Could you check a few things on this model? Use its own coordinates, in mm. A direction names the side the tool comes from. Give positions to 0.01 mm unless a question says otherwise; leave off trailing zeros. Order: outer loops, then holes, each group sorted by start corner. A loop starts at its lowest first (then second) coordinate and runs counter-clockwise, first axis right, second up. Notation, with made-up numbers: (-29, 57) -> (-20, 57) arc R17 cw to (-20, 81) -> close; hole circle Ø4 at (80.25, 41.5). An arc over 180 degrees is marked (long way). Use one line per item in the form item = value. Start each with the question number.
from build123d import *

# Parameters (mm, degrees)
SKETCH1_W           = 66
SKETCH1_H           = 33
SKETCH1_W_2         = 33
BOSS_EXTRUDE1_DEPTH = 100
SKETCH3_W           = 86
SKETCH3_H           = 86
CUT_EXTRUDE1_DEPTH  = 90
CUT_EXTRUDE2_DEPTH  = 2.5
CUT_EXTRUDE3_DEPTH  = 18.5
SKETCH6_W           = 120.471409441
SKETCH6_H           = 36
CUT_EXTRUDE4_DEPTH  = 5
CUT_EXTRUDE5_DEPTH  = 2.5
CUT_EXTRUDE6_DEPTH  = 10
SKETCH9_W           = 60
SKETCH9_H           = 10
CUT_EXTRUDE7_DEPTH  = 5
SKETCH10_W          = 40
SKETCH10_H          = 10
CUT_EXTRUDE8_DEPTH  = 5
SKETCH11_W          = 50
SKETCH11_H          = 50
CUT_EXTRUDE11_DEPTH = 3
CUT_EXTRUDE12_DEPTH = 10


with BuildPart() as part:
    # Sketch1 → Boss-Extrude1 (new body)
    with BuildSketch(Plane.XY):
        with BuildLine():
            Line((15, 0), (91, 0))
            ThreePointArc((91, 0), (101.606601718, 4.393398282), (106, 15))
            Line((106, 15), (106, 91))
            ThreePointArc((106, 91), (101.606601718, 101.606601718), (91, 106))
            Line((91, 106), (15, 106))
            ThreePointArc((15, 106), (4.393398282, 101.606601718), (0, 91))
            Line((0, 91), (0, 15))
            ThreePointArc((0, 15), (4.393398282, 4.393398282), (15, 0))
        make_face()
        with Locations((53, 31.5)):
            Rectangle(SKETCH1_W, SKETCH1_H, mode=Mode.SUBTRACT)
        with Locations((31.5, 69.5)):
            Rectangle(SKETCH1_W_2, SKETCH1_H, mode=Mode.SUBTRACT)
        with Locations((74.5, 69.5)):
            Rectangle(SKETCH1_W_2, SKETCH1_H, mode=Mode.SUBTRACT)
    extrude(amount=-BOSS_EXTRUDE1_DEPTH)

    # Sketch3 → Cut-Extrude1 (cut)
    with BuildSketch(Plane(origin=(0, 0, -100), x_dir=(-1, 0, 0), z_dir=(0, 0, -1))):
        with Locations((-53, 53)):
            Rectangle(SKETCH3_W, SKETCH3_H)
    extrude(amount=-CUT_EXTRUDE1_DEPTH, mode=Mode.SUBTRACT)

    # Sketch4 → Cut-Extrude2 (cut)
    with BuildSketch(Plane(origin=(0, 106, 0), x_dir=(1, 0, 0), z_dir=(0, 1, 0))):
        with BuildLine():
            Line((45, 43), (61, 43))
            ThreePointArc((61, 43), (62.414213562, 42.414213562), (63, 41))
            Line((63, 41), (63, 17))
            ThreePointArc((63, 17), (62.414213562, 15.585786438), (61, 15))
            Line((61, 15), (45, 15))
            ThreePointArc((45, 15), (43.585786438, 15.585786438), (43, 17))
            Line((43, 17), (43, 41))
            ThreePointArc((43, 41), (43.585786438, 42.414213562), (45, 43))
        make_face()
    extrude(amount=-CUT_EXTRUDE2_DEPTH, mode=Mode.SUBTRACT)

    # Sketch5 → Cut-Extrude3 (cut)
    with BuildSketch(Plane(origin=(0, 103.5, 0), x_dir=(1, 0, 0), z_dir=(0, 1, 0))):
        with BuildLine():
            Line((45, 38), (61, 38))
            ThreePointArc((61, 38), (62.414213562, 38.585786438), (63, 40))
            Line((63, 40), (63, 41))
            ThreePointArc((63, 41), (62.414213562, 42.414213562), (61, 43))
            Line((61, 43), (45, 43))
            ThreePointArc((45, 43), (43.585786438, 42.414213562), (43, 41))
            Line((43, 41), (43, 40))
            ThreePointArc((43, 40), (43.585786438, 38.585786438), (45, 38))
        make_face()
    extrude(amount=-CUT_EXTRUDE3_DEPTH, mode=Mode.SUBTRACT)

    # Sketch6 → Cut-Extrude4 (cut)
    with BuildSketch(Plane.XY.offset(-20)):
        with Locations((51.490660341, 68)):
            Rectangle(SKETCH6_W, SKETCH6_H)
    extrude(amount=-CUT_EXTRUDE4_DEPTH, mode=Mode.SUBTRACT)

    # Sketch7 → Cut-Extrude5 (cut)
    with BuildSketch(Plane(origin=(106, 0, 0), x_dir=(0, 0, -1), z_dir=(1, 0, 0))):
        with BuildLine():
            Line((17, 40), (41, 40))
            ThreePointArc((41, 40), (42.414213562, 39.414213562), (43, 38))
            Line((43, 38), (43, 22))
            ThreePointArc((43, 22), (42.414213562, 20.585786438), (41, 20))
            Line((41, 20), (17, 20))
            ThreePointArc((17, 20), (15.585786438, 20.585786438), (15, 22))
            Line((15, 22), (15, 38))
            ThreePointArc((15, 38), (15.585786438, 39.414213562), (17, 40))
        make_face()
    cut_extrude5 = extrude(amount=-CUT_EXTRUDE5_DEPTH, mode=Mode.SUBTRACT)

    # Sketch8 → Cut-Extrude6 (cut)
    with BuildSketch(Plane(origin=(103.5, 0, 0), x_dir=(0, 0, -1), z_dir=(1, 0, 0))):
        with BuildLine():
            Line((40, 40), (41, 40))
            ThreePointArc((41, 40), (42.414213562, 39.414213562), (43, 38))
            Line((43, 38), (43, 22))
            ThreePointArc((43, 22), (42.414213562, 20.585786438), (41, 20))
            Line((41, 20), (40, 20))
            ThreePointArc((40, 20), (38.585786438, 20.585786438), (38, 22))
            Line((38, 22), (38, 38))
            ThreePointArc((38, 38), (38.585786438, 39.414213562), (40, 40))
        make_face()
    cut_extrude6 = extrude(amount=-CUT_EXTRUDE6_DEPTH, mode=Mode.SUBTRACT)

    # Mirror1: Cut-Extrude5, Cut-Extrude6 across plane
    add(cut_extrude5.mirror(Plane(origin=(53, 0, 0), x_dir=(0, 0, 1), z_dir=(1, 0, 0))), mode=Mode.SUBTRACT)
    add(cut_extrude6.mirror(Plane(origin=(53, 0, 0), x_dir=(0, 0, 1), z_dir=(1, 0, 0))), mode=Mode.SUBTRACT)

    # Sketch9 → Cut-Extrude7 (cut)
    with BuildSketch(Plane.XZ):
        with Locations((53, -20)):
            Rectangle(SKETCH9_W, SKETCH9_H)
        with Locations((53, -90)):
            Rectangle(SKETCH9_W, SKETCH9_H)
    extrude(amount=-CUT_EXTRUDE7_DEPTH, mode=Mode.SUBTRACT)

    # Sketch10 → Cut-Extrude8 (cut)
    with BuildSketch(Plane.XZ.offset(-5)):
        with Locations((53, -20)):
            Rectangle(SKETCH10_W, SKETCH10_H)
        with Locations((53, -90)):
            Rectangle(SKETCH10_W, SKETCH10_H)
    extrude(amount=-CUT_EXTRUDE8_DEPTH, mode=Mode.SUBTRACT)

    # Sketch11 → Cut-Extrude11 (cut)
    with BuildSketch(Plane(origin=(0, 10, 0), x_dir=(1, 0, 0), z_dir=(0, 1, 0))):
        with Locations((53, 55)):
            Rectangle(SKETCH11_W, SKETCH11_H)
    extrude(amount=-CUT_EXTRUDE11_DEPTH, mode=Mode.SUBTRACT)

    # Sketch12 → Cut-Extrude12 (cut)
    with BuildSketch(Plane(origin=(0, 7, 0), x_dir=(1, 0, 0), z_dir=(0, 1, 0))):
        Polygon((38, 80), (68, 80), (78, 70.00000089), (78, 40.00000089), (68, 30), (38, 30), (28, 39.99999911), (28, 69.99999911), align=None)
    extrude(amount=-CUT_EXTRUDE12_DEPTH, mode=Mode.SUBTRACT)


solid = part.part
(1) Which directions (+Z, -Z, +X, -X, +Y, -Y) give clear straight access to the entire face, cutting with the end or side of a thin tool? Please do faces 1 (the flat face through (58, 69, -5)), 2 (the flat face through (73, 7, -20)), 3 (the flat face through (2, 40, -30)).
(2) Imagine slicing it at A-A (y = 82). Write out the boundary of the cut face in (x, z).
(3) Imagine slicing it at D-D (y = 17). Write out the boundary of the cut face in (x, z), plus the area to 3 significant figures.
(4) Imagine slicing it at C-C (z = -7.5). Write out the boundary of the cut face in (x, y).
(5) I'm going to push flat-ended pins straight in: pin 1 Ø1.5 at (y, z) = (7, -18) entering from +X; pin 2 Ø2.5 at (y, z) = (2.5, -89) entering from -X; pin 3 Ø5 at (y, z) = (100.5, -31.5) entering from -X. Where does each tip first touch, or does it pass through?
(6) Please list where these lines run through material, in increasing order: probe 1 along X at (y, z) = (71.5, -72.5); probe 2 along X at (y, z) = (28, -20).
(7) We'd pull the mould along Z, two halves only. Please class faces 4 (the flat face through (20, 31, -5)), 5 (the flat face through (73, 7, -90)): pulls with the +Z half, pulls with the -Z half, needs draft (parallel to the pull), parting line crosses it, or undercut.
(8) Imagine slicing it at B-B (x = 17). Write out the boundary of the cut face in (y, z), plus the area to 3 significant figures.
Calculated:
q1.face_1 = +Z, -Z
q1.face_2 = -Y
q1.face_3 = -X
q2.outline = (0, -100) -> (10, -100) -> (10, -25) -> (0, -25) -> close; (0, -20) -> (10, -20) -> (10, -10) -> (15, -10) -> (15, 0) -> (0, 0) -> close; (48, -10) -> (58, -10) -> (58, 0) -> (48, 0) -> close; (91, -10) -> (96, -10) -> (96, -20) -> (106, -20) -> (106, 0) -> (91, 0) -> close; (96, -100) -> (106, -100) -> (106, -25) -> (96, -25) -> close
q3.outline = (0, -100) -> (10, -100) -> (10, -10) -> (20, -10) -> (20, 0) -> (0, 0) -> close; (86, -10) -> (96, -10) -> (96, -100) -> (106, -100) -> (106, 0) -> (86, 0) -> close
q3.area = 2,200 mm2
q4.outline = (0, 15) arc R15 ccw to (15, 0) -> (91, 0) arc R15 ccw to (106, 15) -> (106, 91) arc R15 ccw to (91, 106) -> (15, 106) arc R15 ccw to (0, 91) -> close; hole (15, 53) -> (48, 53) -> (48, 86) -> (15, 86) -> close; hole (20, 15) -> (86, 15) -> (86, 48) -> (20, 48) -> close; hole (58, 53) -> (91, 53) -> (91, 86) -> (58, 86) -> close
q5.pin_1 = 104.13
q5.pin_2 = 5.08
q5.pin_3 = 1.73
q6.probe_1 = 0 to 10, 96 to 106
q6.probe_2 = 2.5 to 10, 96 to 103.5
q7.face_4 = needs draft
q7.face_5 = undercut
q8.outline = (0, -100) -> (10, -100) -> (10, -10) -> (53, -10) -> (53, 0) -> (0, 0) -> close; (86, -10) -> (96, -10) -> (96, -100) -> (106, -100) -> (106, 0) -> (86, 0) -> close
q8.area = 2,530 mm2
